Verification items for the finished model (mm, model axes). A direction names the side the tool comes from. Coordinates: 2 decimals unless noted, no trailing zeros. Loops run counter-clockwise (first coordinate to the right, second up) from the corner with the lowest first, then second, coordinate; pieces in that order, holes last. Notation, with made-up numbers: (7.5, 46.5) -> (57.5, 46.5) arc R16 ccw to (57.5, 51.5) -> close; hole circle Ø2 at (-25, 76). An arc over 180 degrees is marked (long way). Answer as a JSON object with one key per item and string values. Group by question number.
Q1. Cross-section at B-B on y = 24. Record the boundary of the cut face in (x, z), and give its area (3 significant figures).
Q2. Release check for a two-part mould opening along Z. For faces 5 (the flat face through (8, 15, -10)), 6 (the flat face through (10, 15, -5)), 7 (the flat face through (30, 15, -13)), 8 (the flat face through (5, 15, 0)) record: released by +Z, released by -Z, zero draft, split by the parting line, or undercut.
Q3. Cross-section at D-D on x = 2.5. Record the boundary of the cut face in (y, z).
Q4. Cross-section at C-C on z = -5. Record the boundary of the cut face in (x, y), and give its area (3 significant figures).
Q5. Cross-section at A-A on x = 26. Record the boundary of the cut face in (y, z), and give its area (3 significant figures).
Q6. Scan lines: L1, parallel to Y at x = 7.25, z = -5; L2, parallel to X at y = 26, z = -2.25; L3, parallel to X at y = 27, z = -11.5. Record each from-to range of solid material in increasing order.
Q7. Gauge pin test, flat ends, axial feed: pin 1 Ø1 at (y, z) = (4.5, 1) entering from -X; pin 2 Ø8 at (y, z) = (6, -5) entering from +X; pin 3 Ø5 at (y, z) = (14, -4) entering from +X; pin 4 Ø3 at (y, z) = (20.5, -6) entering from -X. Record the tip position at first contact, or that the pin passes through.
Q8. Set-up check for faces 1 (the flat face through (17, 0, -17)), 2 (the flat face through (35, 15, -5)), 3 (the flat face through (28, 15, -10)), 4 (the cylindrical face through (50.19, 15.96, -2.11)): record each of +Z, -Z, +X, -X, +Y, -Y from which the full face is reachable in a straight line by a thin tool's end or side.
```python
from build123d import *

# Parameters (mm, degrees)
SKETCH1_W               = 30
SKETCH1_H               = 10
BOSS_EXTRUDE1_DEPTH     = 30
CUT_EXTRUDE1_DEPTH      = 55
CUT_EXTRUDE1_DEPTH_BACK = 22
SKETCH2_R               = 2.5
SKETCH3_R               = 2.5
BOSS_EXTRUDE2_DEPTH     = 16


with BuildPart() as part:
    # Sketch1 → Boss-Extrude1 (new body)
    with BuildSketch(Plane(origin=(0, 0, 0), x_dir=(1, 0, 0), z_dir=(0, 1, 0))):
        with Locations((-15, 15)):
            Rectangle(SKETCH1_W, SKETCH1_H)
        Polygon((30, 15), (30, 10), (25, 10), (25, 0), (35, 0), (35, 20), (0, 20), (0, 0), (10, 0), (10, 10), (5, 10), (5, 15), align=None)
        with Locations((50, 15)):
            Rectangle(SKETCH1_W, SKETCH1_H)
    extrude(amount=BOSS_EXTRUDE1_DEPTH)

    # Sketch2 → Cut-Extrude1 (cut, two sides: drawn at the far end of the back side and taken through both)
    with BuildSketch(Plane(origin=(10, 0, 0), x_dir=(0, 0, -1), z_dir=(1, 0, 0)).offset(-CUT_EXTRUDE1_DEPTH_BACK)):
        with Locations(Location((5, 24, 0), (0, 0, 180))):
            Circle(SKETCH2_R)
        with Locations(Location((5, 6, 0), (0, 0, 180))):
            Circle(SKETCH2_R)
    extrude(amount=CUT_EXTRUDE1_DEPTH + CUT_EXTRUDE1_DEPTH_BACK, mode=Mode.SUBTRACT)

    # Sketch3 → Boss-Extrude2 (add)
    with BuildSketch(Plane.XY.offset(-10)):
        with Locations((-17.5, 15)):
            Circle(SKETCH3_R)
        with Locations(Location((52.5, 15, 0), (0, 0, 180))):
            Circle(SKETCH3_R)
    extrude(amount=BOSS_EXTRUDE2_DEPTH)


solid = part.part
```
Computed values:
{
 "1": {"outline": "(-30, -20) -> (65, -20) -> (65, -10) -> (35, -10) -> (35, -7.5) -> (25, -7.5) -> (25, -10) -> (30, -10) -> (30, -15) -> (5, -15) -> (5, -10) -> (10, -10) -> (10, -7.5) -> (0, -7.5) -> (0, -10) -> (-30, -10) -> close; (0, -2.5) -> (10, -2.5) -> (10, 0) -> (0, 0) -> close; (25, -2.5) -> (35, -2.5) -> (35, 0) -> (25, 0) -> close", "area": "925 mm²"},
 "2": {"face 5": "undercut", "face 6": "zero draft", "face 7": "undercut", "face 8": "released by +Z"},
 "3": {"outline": "(0, -20) -> (30, -20) -> (30, 0) -> (0, 0) -> close; hole circle Ø5 at (6, -5); hole circle Ø5 at (24, -5)"},
 "4": {"outline": "circle Ø5 at (-17.5, 15); (0, 0) -> (10, 0) -> (10, 3.5) -> (0, 3.5) -> close; (0, 8.5) -> (10, 8.5) -> (10, 21.5) -> (0, 21.5) -> close; (0, 26.5) -> (10, 26.5) -> (10, 30) -> (0, 30) -> close; (25, 0) -> (35, 0) -> (35, 3.5) -> (25, 3.5) -> close; (25, 8.5) -> (35, 8.5) -> (35, 21.5) -> (25, 21.5) -> close; (25, 26.5) -> (35, 26.5) -> (35, 30) -> (25, 30) -> close; circle Ø5 at (52.5, 15)", "area": "439 mm²"},
 "5": {"outline": "(0, -20) -> (30, -20) -> (30, -15) -> (0, -15) -> close; (0, -10) -> (30, -10) -> (30, 0) -> (0, 0) -> close; hole circle Ø5 at (6, -5); hole circle Ø5 at (24, -5)", "area": "411 mm²"},
 "6": {"L1": "y = 0 to 3.5, 8.5 to 21.5, 26.5 to 30", "L2": "x = 0 to 10, 25 to 35", "L3": "x = -30 to 5, 30 to 65"},
 "7": {"pin 1": "passes through", "pin 2": "stops at x = 35", "pin 3": "stops at x = 55", "pin 4": "stops at x = 0"},
 "8": {"face 1": "+Z, -Z, +X, -X, -Y", "face 2": "+Z, +Y, -Y", "face 3": "+Y, -Y", "face 4": "+Z"}
}
